```python
from build123d import *

# Parameters (mm, degrees)
CUT_EXTRUDE_1_DEPTH = 1.8


with BuildPart() as part:
    # 草图1 → 旋转1 (revolve)
    with BuildSketch(Plane.XY, mode=Mode.PRIVATE) as revolve_1_sk:
        Polygon((0, 0), (0, 2.35), (2, 2.35), (2, 3.35), (7, 3.35), (7, 3.85), (31, 3.85), (31, 4.85), (51, 4.85), (51, 3.85), (59, 3.85), (59, 3.35), (64, 3.35), (64, 2.35), (66, 2.35), (66, 0), align=None)
    revolve(revolve_1_sk.sketch.rotate(Axis((0, 0, 0), (1, 0, 0)), 180), axis=Axis((0, 0, 0), (1, 0, 0)))

    # 草图2 → 切除-拉伸1 (cut)
    with BuildSketch(Plane.XY.offset(3.85)):
        with BuildLine():
            Line((25.5, 1.5), (28.5, 1.5))
            ThreePointArc((28.5, 1.5), (30, 0), (28.5, -1.5))
            Line((28.5, -1.5), (25.5, -1.5))
            ThreePointArc((25.5, -1.5), (24, 0), (25.5, 1.5))
        make_face()
        with BuildLine():
            Line((53.5, 1.5), (56.5, 1.5))
            ThreePointArc((56.5, 1.5), (58, 0), (56.5, -1.5))
            Line((56.5, -1.5), (53.5, -1.5))
            ThreePointArc((53.5, -1.5), (52, 0), (53.5, 1.5))
        make_face()
    extrude(amount=-CUT_EXTRUDE_1_DEPTH, mode=Mode.SUBTRACT)


solid = part.part
```
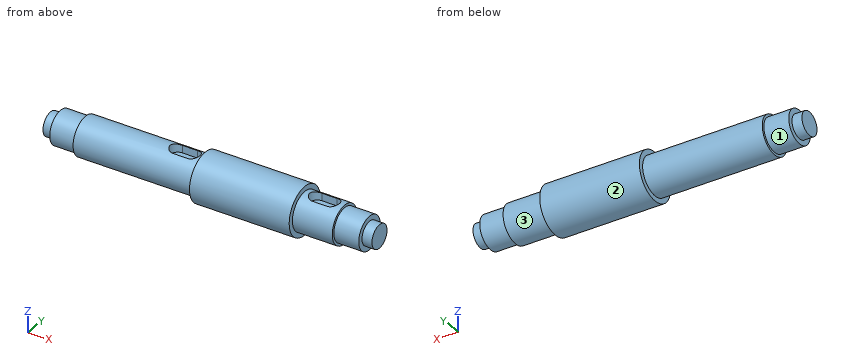
The listing builds one solid part. Answer for the finished solid, in the listing's coordinates (mm). Face numbers are marked on the shaded views. A direction names the side the tool comes from. Give positions to 0.01 mm unless a question says otherwise; leave off trailing zeros. Order: outer loops, then holes, each group sorted by start corner. A loop starts at its lowest first (then second) coordinate and runs counter-clockwise, first axis right, second up.
Item 1: The part is cut by section A-A, the plane z = 0.75. Give the vertices of the cut face in (x, y), and give its area (3 significant figures).
From the geometry:
outline: (0, -2.23) - (2, -2.23) - (2, -3.26) - (7, -3.26) - (7, -3.78) - (31, -3.78) - (31, -4.79) - (51, -4.79) - (51, -3.78) - (59, -3.78) - (59, -3.26) - (64, -3.26) - (64, -2.23) - (66, -2.23) - (66, 2.23) - (64, 2.23) - (64, 3.26) - (59, 3.26) - (59, 3.78) - (51, 3.78) - (51, 4.79) - (31, 4.79) - (31, 3.78) - (7, 3.78) - (7, 3.26) - (2, 3.26) - (2, 2.23) - (0, 2.23) - close
area: 516 mm2
Item 2: Find the intervals of material crossed by probe 1 along X at (y, z) = (0, -2.5); probe 2 along Y at (x, z) = (28, 2.75); probe 3 along Z at (x, y) = (43.5, -0.25), in increasing order.
From the geometry:
probe 1: x = 2 to 64
probe 2: y = -2.69 to -1.5, 1.5 to 2.69
probe 3: z = -4.84 to 4.84
Item 3: The part is cut by section B-B, the plane x = 22.5. Give the vertices of the cut face in (y, z), and give its area (3 significant figures).
From the geometry:
outline: circle Ø7.7 at (0, 0)
area: 46.6 mm2
Item 4: The part is cut by section C-C, the plane x = 43. Give the vertices of the cut face in (y, z), and give its area (3 significant figures).
From the geometry:
outline: circle Ø9.7 at (0, 0)
area: 73.9 mm2
Item 5: Which of the six approach directions +Z, -Z, +X, -X, +Y, -Y give full straight-line access (tool end or side, diameter ignored) to the marked faces 1, 2 and 3?
From the geometry:
face 1: -X
face 2: +X, -X
face 3: +X
Item 6: Given pin 1 Ø3 at (x, y) = (25.5, 2) entering from -Z; pin 2 Ø0.7 at (x, z) = (54.5, 2.5) entering from +Y; pin 3 Ø1.5 at (x, y) = (26, 0) entering from +Z, each flat-ended and moving along its own axis, determine where each tip first touches the part or whether it passes through.
From the geometry:
pin 1: stops at z = -3.82
pin 2: stops at y = 3.19
pin 3: stops at z = 2.05
